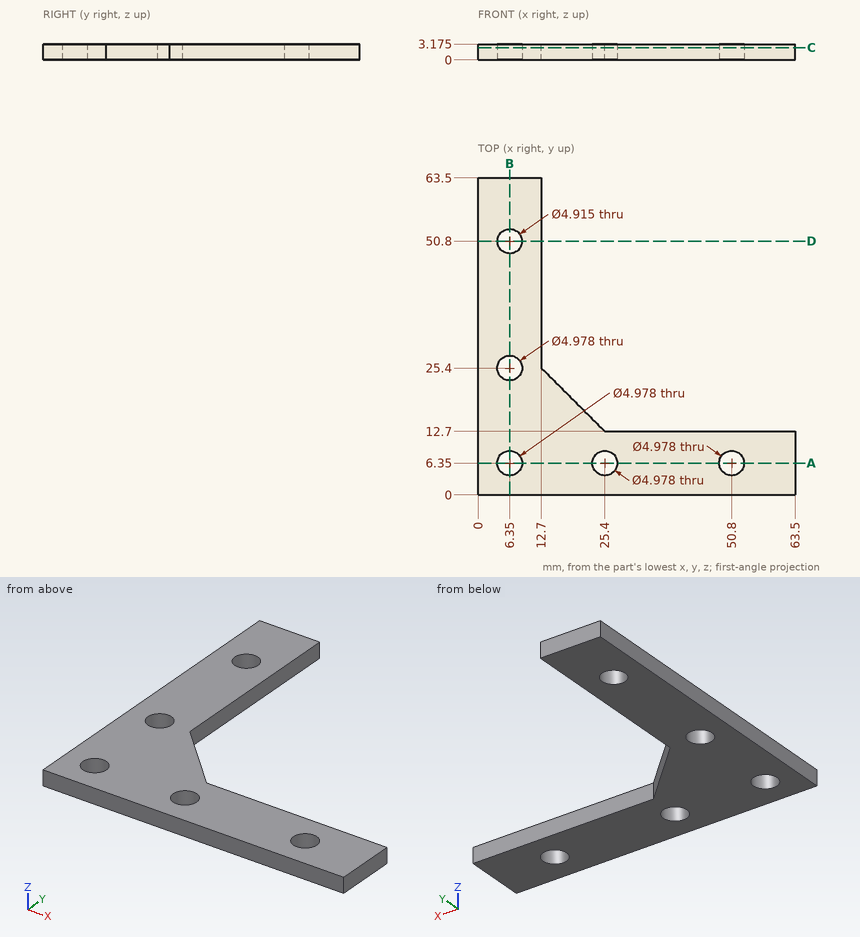
For this review, use the dimensioned drawing (mm, ordinates from the lowest corner) and the shaded views. Round coordinates to 2 decimals unless told otherwise and drop trailing zeros. Write each loop counter-clockwise with the first axis right and the second up, starting at its lowest first coordinate (ties: lowest second). Pieces come first, ordered by that corner, then holes. Notation, with made-up numbers: (80, -3.5) -> (133, -3.5) arc R21 cw to (133, 35.5) -> close; hole circle Ø11 at (-23.5, 33.25). An arc over 180 degrees is marked (long way). Answer in a Markdown table with one row per item.
Q1. Take a section at D-D, the plane y = 50.8. State the section outline as (x, z) points (1 decimal), then the cut area to 3 significant figures.
The answers:
| item | result |
|---|---|
| outline | (0, 0) -> (3.9, 0) -> (3.9, 3.2) -> (0, 3.2) -> close; (8.8, 0) -> (12.7, 0) -> (12.7, 3.2) -> (8.8, 3.2) -> close |
| area | 24.7 mm² |
Q2. Take a section at C-C, the plane z = 2.45. Count the separate pieces of the cut face and the enclosed holes in it, then the cut area to 3 significant figures.
The answers:
| item | result |
|---|---|
| separate pieces | 1 |
| enclosed holes | 5 |
| area | 1,440 mm² |
Q3. Take a section at A-A, the plane y = 6.35. State the section outline as (x, z) points (1 decimal), then the cut area to 3 significant figures.
The answers:
| item | result |
|---|---|
| outline | (0, 0) -> (3.9, 0) -> (3.9, 3.2) -> (0, 3.2) -> close; (8.8, 0) -> (22.9, 0) -> (22.9, 3.2) -> (8.8, 3.2) -> close; (27.9, 0) -> (48.3, 0) -> (48.3, 3.2) -> (27.9, 3.2) -> close; (53.3, 0) -> (63.5, 0) -> (63.5, 3.2) -> (53.3, 3.2) -> close |
| area | 154 mm² |
Q4. To check wall thickness, follow L1, parallel to Y at x = 6.35, z = 1.3; L2, parallel to Y at x = 50.8, z = 1.9; L3, parallel to X at y = 56.5, z = 0.75. State the ranges of each line that lie inside material, in increasing order. Write a range as [from, to].
The answers:
| item | result |
|---|---|
| L1 | [0, 3.86], [8.84, 22.91], [27.89, 48.34], [53.26, 63.5] |
| L2 | [0, 3.86], [8.84, 12.7] |
| L3 | [0, 12.7] |
Q5. Clearance check with flat-ended pins moving along their axes: pin 1 Ø1 at (x, z) = (54, 1) entering from +Y; pin 2 Ø1.5 at (y, z) = (55, 1) entering from +X. State where each tip first meets the part, or that it passes through.
The answers:
| item | result |
|---|---|
| pin 1 | y = 12.7 |
| pin 2 | x = 12.7 |
